Autodesk Fusion 360 part; units mm, degrees
sketch "Sketch1" plane through (0, 0, 0) normal (0, 0, 1) x (1, 0, 0)
  line L0 (0, 0) -> (76, 0)
  line L1 (76, 0) -> (76, 112)
  line L2 (76, 112) -> (0, 112)
  line L3 (0, 112) -> (0, 0)
  circle A0 centre (4.75, 96.5) radius 2
  circle A1 centre (71.25, 96.5) radius 2
  circle A2 centre (71.25, 6.5) radius 2
  circle A3 centre (4.75, 6.5) radius 2
  line L4 (4.75, 96.5) -> (71.25, 96.5) construction
  line L5 (71.25, 96.5) -> (71.25, 6.5) construction
  line L6 (38, 112) -> (38, 0) construction
  dimension "d1" = 76
  dimension "d2" = 112
  dimension "d3" = 66.5
  dimension "d4" = 90
  dimension "d5" = 66.5
  dimension "d6" = 90
  dimension "d7" = 4
  dimension "d8" = 4
  dimension "d9" = 4
  dimension "d10" = 4
  dimension "d11" = 6.5
extrude "Extrude1" add sketch "Sketch1" along normal blind 6
sketch "Sketch2" plane through (0, 0, 0) normal (0, 0, -1) x (1, 0, 0)
  circle A0 centre (71.25, -96.5) radius 2
  circle A1 centre (4.75, -96.5) radius 2
  circle A2 centre (71.25, -6.5) radius 2
  circle A3 centre (4.75, -6.5) radius 2
  line L0 (0, 0) -> (0, -112)
  line L1 (0, -112) -> (76, -112)
  line L2 (76, -112) -> (76, 0)
  line L3 (76, 0) -> (0, 0)
  line L4 (76, -112) -> (0, -112)
  line L5 (0, -112) -> (0, -105.5)
  line L6 (0, -105.5) -> (76, -105.5)
  line L7 (76, -105.5) -> (76, -112)
  dimension "d14" = 6.5
extrude "Extrude2" add sketch "Sketch2" along normal blind 14 contours L0 L1 L2 L4 L5 L6 L7
ref_plane "WorkPlane1" through (53, 56, -4) normal (1, 0, 0) x (0, 1, 0)
sketch "Sketch3" plane through (53, 56, -4) normal (1, 0, 0) x (0, 1, 0)
  line L0 (-56, 4) -> (49.5, 4)
  line L1 (49.5, 4) -> (49.5, -10)
  line L2 (49.5, -10) -> (56, -10)
  line L3 (56, -10) -> (56, 10)
  line L4 (56, 10) -> (-56, 10)
  line L5 (-56, 10) -> (-56, 4)
  line L6 (-56, 4) -> (49.5, 4)
  line L7 (49.5, -10) -> (-27.892, 4)
extrude "Extrude3" add sketch "Sketch3" along normal mid plane 6 contours L0 L1 L6 L7
ref_plane "WorkPlane2" through (23, 56, -4) normal (-1, 0, 0) x (0, -1, 0)
sketch "Sketch4" plane through (23, 56, -4) normal (-1, 0, 0) x (0, 1, 0)
  line L0 (49.5, -4) -> (49.5, 10)
  line L1 (49.5, 10) -> (-27.892, -4)
  line L2 (-27.892, -4) -> (49.5, -4)
  line L3 (49.5, 10) -> (-27.892, -4)
extrude "Extrude4" add sketch "Sketch4" along normal mid plane 6
sketch "Sketch5" plane through (0, 112, 0) normal (0, 1, 0) x (-1, 0, 0)
  line L0 (0, -14) -> (0, 6)
  line L1 (0, 6) -> (-76, 6)
  line L2 (-76, 6) -> (-76, -14)
  line L3 (-76, -14) -> (0, -14)
  circle A0 centre (-67.21, -8.5) radius 2
  line L4 (-38, 6) -> (-38, -14) construction
  circle A1 centre (-8.79, -8.5) radius 2
  dimension "d23" = 4
  dimension "d24" = 4
  dimension "d25" = 58.42
  dimension "d26" = 5.5
extrude "Extrude5" cut sketch "Sketch5" against normal blind 6.5 contours A0 | A1
fillet "Fillet1" radius 4 2 edges at (76, 0, 3) (0, 0, 3)
fillet "Fillet2" radius 3 2 edges at (0, 108.75, -14) (76, 108.75, -14)
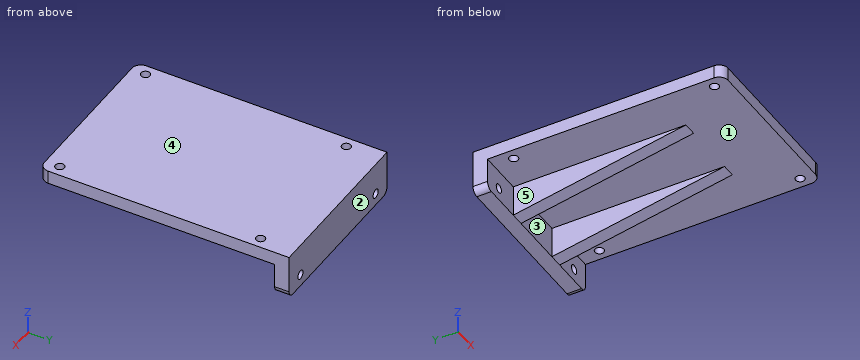
Input: part model. Units: mm. Frame: model coordinates. Face numbers are marked on the shaded views. A direction names the side the tool comes from. Give positions to 0.01 mm unless a question says otherwise; leave off trailing zeros. Order: outer loops, then holes, each group sorted by start corner. A loop starts at its lowest first (then second) coordinate and runs counter-clockwise, first axis right, second up. Notation, with made-up numbers: (85, 23.25) - (99, 23.25) arc R24 cw to (99, 43.25) - close; hole circle Ø4 at (6, 6.5). An arc over 180 degrees is marked (long way). Use a Markdown table: item, result.
(1) Section query A-A (x = 67.21). Output: boundary loops of the cut face in (y, z).
Computed values:
| item | result |
|---|---|
| outline | (0, 0) - (105.5, 0) - (105.5, -6.5) - (112, -6.5) - (112, 6) - (0, 6) - close; (105.5, -14) - (112, -14) - (112, -10.5) - (105.5, -10.5) - close |
(2) Pin query (flat end, axial travel): pin 1 (11 mm diameter, centred on y = 60, z = -10.5, fed in from -X); pin 2 (4 mm diameter, centred on x = 61.5, z = -5, fed in from -Y); pin 3 (4 mm diameter, centred on y = 64, z = -5.5, fed in from +X). Return the tip coordinate at first contact, or that it passes through.
Computed values:
| item | result |
|---|---|
| pin 1 | stops at x = 20 |
| pin 2 | stops at y = 105.5 |
| pin 3 | stops at x = 56 |
(3) Draft query along X for the marked faces 3, 4 and 5. Return one class per face: released by +X, released by -X, zero draft, split by the parting line, or undercut.
Computed values:
| item | result |
|---|---|
| face 3 | undercut |
| face 4 | zero draft |
| face 5 | released by -X |
(4) Line query: line 1 (Y direction, x = 4.75, z = 1.65); line 2 (Z direction, x = 8.79, y = 109.75); line 3 (X direction, y = 58, z = -3.5). Output: solid intervals per line, ascending. Write a range as from..to.
Computed values:
| item | result |
|---|---|
| line 1 | y = 0..4.5, 8.5..94.5, 98.5..112 |
| line 2 | z = -14..-10.5, -6.5..6 |
| line 3 | x = 20..26, 50..56 |
(5) Section query B-B (y = 6.5). Output: boundary loops of the cut face in (x, z), then the cut area to 3 significant figures.
Computed values:
| item | result |
|---|---|
| outline | (0, 0) - (2.75, 0) - (2.75, 6) - (0, 6) - close; (6.75, 0) - (69.25, 0) - (69.25, 6) - (6.75, 6) - close; (73.25, 0) - (76, 0) - (76, 6) - (73.25, 6) - close |
| area | 408 mm2 |
(6) Access query for the marked faces 1 and 2. Directions: +Z, -Z, +X, -X, +Y, -Y. A direction counts if a zero-diameter tool reaches every point of the face in a straight line with its end or side. Return the directions, or none.
Computed values:
| item | result |
|---|---|
| face 1 | -Z, -Y |
| face 2 | +Z, -Z, +X, -X, +Y |
(7) Section query C-C (z = -3.25). Output: boundary loops of the cut face in (x, y), then the cut area to 3 significant figures.
Computed values:
| item | result |
|---|---|
| outline | (0, 105.5) - (20, 105.5) - (20, 46.07) - (26, 46.07) - (26, 105.5) - (50, 105.5) - (50, 46.07) - (56, 46.07) - (56, 105.5) - (76, 105.5) - (76, 112) - (0, 112) - close |
| area | 1,210 mm2 |
(8) Section query D-D (y = 31). Output: boundary loops of the cut face in (x, z).
Computed values:
| item | result |
|---|---|
| outline | (0, 0) - (20, 0) - (20, -0.52) - (26, -0.52) - (26, 0) - (50, 0) - (50, -0.52) - (56, -0.52) - (56, 0) - (76, 0) - (76, 6) - (0, 6) - close |
